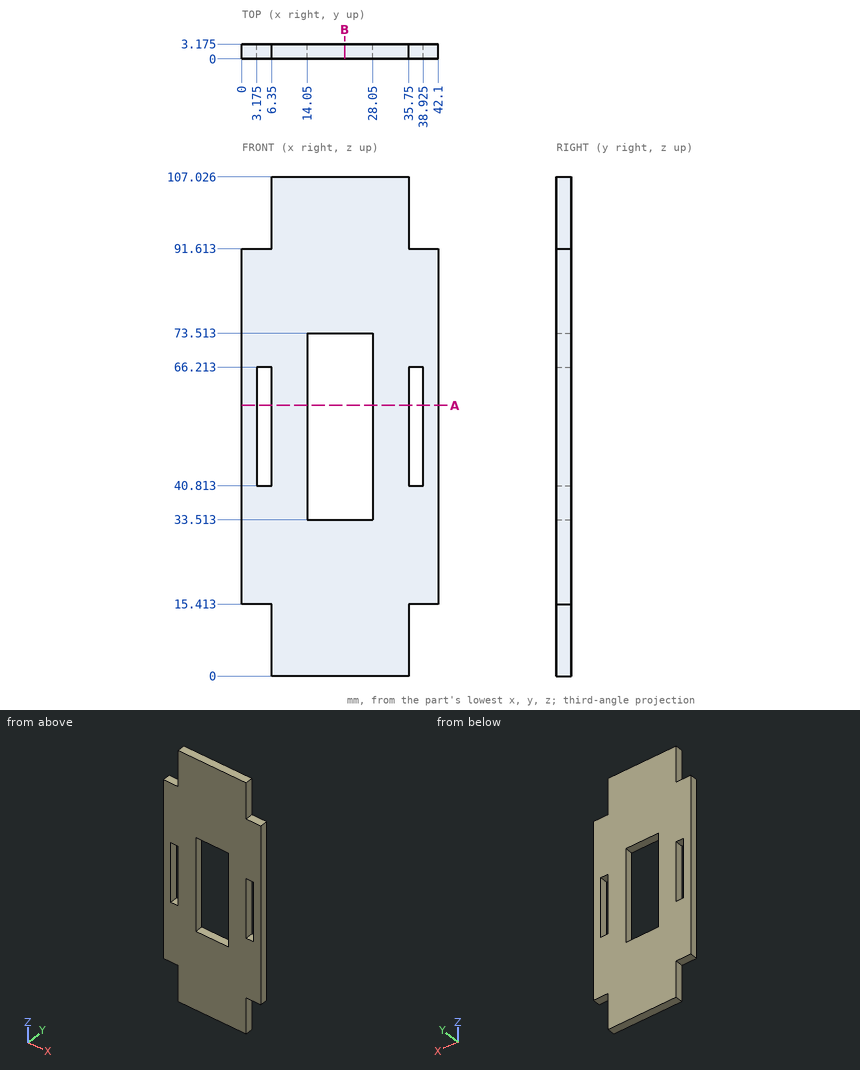
The figure shows three views and two pictorial views of one solid part (mm, origin at its lowest corner). Answer the questions. Give positions to 0.01 mm unless a question says otherwise; leave off trailing zeros. Order: outer loops, then holes, each group sorted by start corner. A loop starts at its lowest first (then second) coordinate and runs counter-clockwise, first axis right, second up. Notation, with made-up numbers: M 45,86 L 68,86 A34 ccw 68,123 Z; hole C 33,68.25 d9. An arc over 180 degrees is marked long. Return JSON: item names as keys, results as strings.
1) Straight lines are drawn through the part: line 1 along Z through (x, y) = (20.5, 2.9); line 2 along X through (y, z) = (0.45, 67.5); line 3 along Z through (x, y) = (37, 1.7). For each, find the intervals that lie inside material, in ascending order. Write a range as [from, to].
Resolved:
{"line 1": "[0, 33.51], [73.51, 107.03]", "line 2": "[0, 14.05], [28.05, 42.1]", "line 3": "[15.41, 40.81], [66.21, 91.61]"}
2) Section B-B, the plane x = 22 is taken. Write down the section's boundary in (y, z) (1 decimal), plus the area to 3 significant figures.
Resolved:
{"outline": "M 0,0 L 3.2,0 L 3.2,33.5 L 0,33.5 Z; M 0,73.5 L 3.2,73.5 L 3.2,107 L 0,107 Z", "area": "213 mm^2"}
3) Each of these flat-tipped pins is pushed along its axis until it touches: pin 1 (1.6 mm diameter, centred on y = 1.5, z = 10, fed in from +X); pin 2 (1.6 mm diameter, centred on x = 37, y = 2, fed in from +Z); pin 3 (1.6 mm diameter, centred on y = 1.5, z = 98.5, fed in from -X). Where does it stop, or does it pass through?
Resolved:
{"pin 1": "x = 35.75", "pin 2": "z = 91.61", "pin 3": "x = 6.35"}
4) Section A-A, the plane z = 58 is taken. Give the number of separate pieces and of enclosed holes in the cut face.
Resolved:
{"separate pieces": "4", "enclosed holes": "0"}
